```python
from build123d import *

# Parameters (mm, degrees)
SKETCH1_W               = 47
SKETCH1_H               = 47
BOSS_EXTRUDE1_DEPTH     = 4
CUT_EXTRUDE1_DEPTH      = 34.473870407
CUT_EXTRUDE1_DEPTH_BACK = 34.473870407
CUT_EXTRUDE2_DEPTH      = 34.473870407
CUT_EXTRUDE2_DEPTH_BACK = 34.473870407
SKETCH3_R               = 2.5
SKETCH4_W               = 47
SKETCH4_H               = 47
SKETCH4_W_2             = 43
SKETCH4_H_2             = 43
BOSS_EXTRUDE2_DEPTH     = 8
SKETCH5_W               = 2
SKETCH5_H               = 5.263518928
CUT_EXTRUDE3_DEPTH      = 5


with BuildPart() as part:
    # Sketch1 → Boss-Extrude1 (new body)
    with BuildSketch(Plane.XY):
        Rectangle(SKETCH1_W, SKETCH1_H)
    extrude(amount=BOSS_EXTRUDE1_DEPTH)

    # Sketch2 → Cut-Extrude1 (cut, two sides: drawn at the far end of the back side and taken through both)
    with BuildSketch(Plane.XY.offset(4).offset(-CUT_EXTRUDE1_DEPTH_BACK)):
        with BuildLine():
            Line((-2.2, 1.187434209), (-2.2, -1.187434209))
            ThreePointArc((-2.2, -1.187434209), (0, -2.5), (2.2, -1.187434209))
            Line((2.2, -1.187434209), (2.2, 1.187434209))
            ThreePointArc((2.2, 1.187434209), (0, 2.5), (-2.2, 1.187434209))
        make_face()
    extrude(amount=CUT_EXTRUDE1_DEPTH + CUT_EXTRUDE1_DEPTH_BACK, mode=Mode.SUBTRACT)

    # Sketch3 → Cut-Extrude2 (cut, two sides: drawn at the far end of the back side and taken through both)
    with BuildSketch(Plane.XY.offset(4).offset(-CUT_EXTRUDE2_DEPTH_BACK)):
        with Locations((-17.5, 17.5)):
            Circle(SKETCH3_R)
    extrude(amount=CUT_EXTRUDE2_DEPTH + CUT_EXTRUDE2_DEPTH_BACK, mode=Mode.SUBTRACT)

    # Sketch4 → Boss-Extrude2 (add)
    with BuildSketch(Plane.XY.offset(4)):
        Rectangle(SKETCH4_W, SKETCH4_H)
        Rectangle(SKETCH4_W_2, SKETCH4_H_2, mode=Mode.SUBTRACT)
    extrude(amount=BOSS_EXTRUDE2_DEPTH)

    # Sketch5 → Cut-Extrude3 (cut)
    with BuildSketch(Plane.XY.offset(12)):
        with Locations((22.5, 0)):
            Rectangle(SKETCH5_W, SKETCH5_H)
    extrude(amount=-CUT_EXTRUDE3_DEPTH, mode=Mode.SUBTRACT)


solid = part.part
```
Build history of the part. All positions in model axes, mm. A direction names the side the tool comes from. Coordinates: 2 decimals unless noted, no trailing zeros. Order: outer loops, then holes, each group sorted by start corner. A loop starts at its lowest first (then second) coordinate and runs counter-clockwise, first axis right, second up.
Item 1: Tool access for faces 1 (the flat face through (0, -5, 0)), 2 (the flat face through (-2.2, 0, 2)), 3 (the flat face through (22, 0, 7)), 4 (the flat face through (21.5, 0, 6)): list every direction of +Z, -Z, +X, -X, +Y, -Y with a clear straight run to the whole face (end or side of a thin tool).
Filled in:
face 1: -Z, +X, -X, +Y, -Y
face 2: +Z, -Z
face 3: +Z, +X
face 4: +Z
Item 2: Saw through at A-A on x = 1.5. List the corners of the cut face in (y, z).
Filled in:
outline: (-23.5, 0) - (-2, 0) - (-2, 4) - (-21.5, 4) - (-21.5, 12) - (-23.5, 12) - close; (2, 0) - (23.5, 0) - (23.5, 12) - (21.5, 12) - (21.5, 4) - (2, 4) - close
Item 3: Saw through at B-B on z = 1.25. List the corners of the cut face in (x, y), then the cut area to 3 significant figures.
Filled in:
outline: (-23.5, -23.5) - (23.5, -23.5) - (23.5, 23.5) - (-23.5, 23.5) - close; hole circle Ø5 at (-17.5, 17.5); hole (-2.2, -1.19) arc R2.5 ccw to (2.2, -1.19) - (2.2, 1.19) arc R2.5 ccw to (-2.2, 1.19) - close
area: 2,170 mm2
Item 4: Saw through at C-C on y = 17.5. List the corners of the cut face in (x, z), then the cut area to 3 significant figures.
Filled in:
outline: (-23.5, 0) - (-20, 0) - (-20, 4) - (-21.5, 4) - (-21.5, 12) - (-23.5, 12) - close; (-15, 0) - (23.5, 0) - (23.5, 12) - (21.5, 12) - (21.5, 4) - (-15, 4) - close
area: 200 mm2
Item 5: Drill centre lines: L1, parallel to Y at x = -11, z = 8; L2, parallel to X at y = 17.5, z = 2.95. Where is each one in solid material? Low to high.
Filled in:
L1: y = -23.5 to -21.5, 21.5 to 23.5
L2: x = -23.5 to -20, -15 to 23.5
Item 6: Saw through at D-D on z = 5.5. List the corners of the cut face in (x, y).
Filled in:
outline: (-23.5, -23.5) - (23.5, -23.5) - (23.5, 23.5) - (-23.5, 23.5) - close; hole (-21.5, -21.5) - (21.5, -21.5) - (21.5, 21.5) - (-21.5, 21.5) - close
Item 7: Drop flat-ended pins along their axis: pin 1 Ø21.5 at (x, y) = (3.5, -0.5) entering from +Z; pin 2 Ø1.6 at (x, y) = (22.5, 0) entering from +Z. Give the stop position or say it passes through.
Filled in:
pin 1: stops at z = 4
pin 2: stops at z = 7
Item 8: Mould opens along Y. For faces 5 (the flat face through (-23, 0, 12)), 6 (the flat face through (4, 0, 4)), 7 (the flat face through (0, -23.5, 6)), 8 (the flat face through (0, 23.5, 6)) say: released by +Y, released by -Y, zero draft, split by the parting line, or undercut.
Filled in:
face 5: zero draft
face 6: undercut
face 7: released by -Y
face 8: released by +Y
